For this review, take the finished solid that the model builds, in its own axes (mm). A direction names the side the tool comes from. Round coordinates to 2 decimals unless told otherwise and drop trailing zeros. Write each loop counter-clockwise with the first axis right and the second up, starting at its lowest first coordinate (ties: lowest second). Pieces come first, ordered by that corner, then holes. Notation, with made-up numbers: M 55,61.25 L 83,61.25 A16 cw 83,66.25 Z; hole C -36.5,32.25 d5. An arc over 180 degrees is marked long. Write each question's results on one line, items separated by ' | '. Start each with the question number.
```python
from build123d import *

# Parameters (mm, degrees)
SKETCH5_W           = 500
SKETCH5_H           = 200
BOSS_EXTRUDE2_DEPTH = 200
SHELL2_T            = -20
SKETCH6_R           = 26.25
SKETCH6_W           = 51.5
SKETCH6_H           = 51.5
CUT_EXTRUDE2_DEPTH  = 51.6


with BuildPart() as part:
    # Sketch5 → Boss-Extrude2 (new body)
    with BuildSketch(Plane.XY):
        Rectangle(SKETCH5_W, SKETCH5_H)
    extrude(amount=BOSS_EXTRUDE2_DEPTH)

    # Shell2
    shell2_openings = [part.faces().sort_by_distance(p)[0] for p in [
        (0, 0, 0),
    ]]
    offset(amount=SHELL2_T, openings=shell2_openings, kind=Kind.INTERSECTION)

    # Sketch6 → Cut-Extrude2 (cut)
    with BuildSketch(Plane.XY.offset(200)):
        with Locations((-150, 0)):
            Circle(SKETCH6_R)
        Polygon((14.866769432, 25.75), (-14.866769432, 25.75), (-29.733538863, 0), (-14.866769432, -25.75), (14.866769432, -25.75), (29.733538863, 0), align=None)
        with Locations((150, 0)):
            Rectangle(SKETCH6_W, SKETCH6_H)
    extrude(amount=-CUT_EXTRUDE2_DEPTH, mode=Mode.SUBTRACT)


solid = part.part
```
Item 1: For faces 5 (the flat face through (175.75, 0, 190)), 6 (the flat face through (-3, 37, 180)), 7 (the flat face through (250, -1, 99)), list the 3-axis set-ups (+Z, -Z, +X, -X, +Y, -Y) from which the entire face can be reached by the end or side of a thin tool; tool diameter is ignored.
Item 2: We need section A-A on x = -150. State the section outline as (y, z) points.
Item 3: We need section B-B on y = 12. State the section outline as (x, z) points.
Item 4: For probe 1 along Y at (x, z) = (122, 92); probe 2 along X at (y, z) = (68, 22); probe 3 along Y at (x, z) = (-150, 190.5), list the stretches that pass through material, from the lowest coordinate up.
Item 5: Insertion check: P1, Ø1, axis at x = 74, y = -58, coming from the -Z side. The pin has a flat end and moves straight along its axis. Give the tip position at first contact, or say it passes through.
Item 6: We need section C-C on z = 148. State the section outline as (x, y) points, then the cut area to 3 significant figures.
Item 7: We need section D-D on y = -62. State the section outline as (x, z) points.
Item 8: Mouldability with a two-part tool opening along Y and no side actions: class faces 1 (the flat face through (230, -1, 89)), 2 (the flat face through (-3, -100, 99)), 3 (the flat face through (-20, -81, 0)), 4 (the cylindrical face through (-125, 8, 190)) as pulls with the +Y half, pulls with the -Y half, needs draft (parallel to the pull), parting line crosses it, or undercut.
Numbers:
1) face 5: +Z, -Z | face 6: -Z | face 7: +Z, -Z, +X, +Y, -Y
2) outline: M -100,0 L -80,0 L -80,180 L -26.25,180 L -26.25,200 L -100,200 Z; M 26.25,180 L 80,180 L 80,0 L 100,0 L 100,200 L 26.25,200 Z
3) outline: M -250,0 L -230,0 L -230,180 L -173.35,180 L -173.35,200 L -250,200 Z; M -126.65,180 L -22.81,180 L -22.81,200 L -126.65,200 Z; M 22.81,180 L 124.25,180 L 124.25,200 L 22.81,200 Z; M 175.75,180 L 230,180 L 230,0 L 250,0 L 250,200 L 175.75,200 Z
4) probe 1: y = -100 to -80, 80 to 100 | probe 2: x = -250 to -230, 230 to 250 | probe 3: y = -100 to -26.25, 26.25 to 100
5) P1: stops at z = 180
6) outline: M -250,-100 L 250,-100 L 250,100 L -250,100 Z; hole M -230,-80 L 230,-80 L 230,80 L -230,80 Z | area: 26,400 mm^2
7) outline: M -250,0 L -230,0 L -230,180 L 230,180 L 230,0 L 250,0 L 250,200 L -250,200 Z
8) face 1: undercut | face 2: pulls with the -Y half | face 3: needs draft | face 4: undercut
